Autodesk Inventor part; units mm, degrees
ref_plane "YZ Plane" through (0, 0, 0) normal (1, 0, 0) x (0, 1, 0)
ref_plane "XZ Plane" through (0, 0, 0) normal (0, 1, 0) x (-1, 0, 0)
ref_plane "XY Plane" through (0, 0, 0) normal (0, 0, 1) x (1, 0, 0)
sketch "Sketch1" plane through (0, 0, 0) normal (0, 0, 1) x (1, 0, 0)
  circle A0 centre (0, 0) radius 6.35
  line L0 (0, 10.9985) -> (9.525, 5.4993)
  line L1 (9.525, 5.4993) -> (9.525, -5.4993)
  line L2 (9.525, -5.4993) -> (0, -10.9985)
  line L3 (0, -10.9985) -> (-9.525, -5.4993)
  line L4 (-9.525, -5.4993) -> (-9.525, 5.4993)
  line L5 (-9.525, 5.4993) -> (0, 10.9985)
  dimension "d1" = 19.05
extrude "Extrusion1" add sketch "Sketch1" against normal blind 12.7 contours A0 | L0 L1 L2 L3 L4 L5
sketch "Sketch2" plane through (0, 0, 0) normal (0, 0, 1) x (1, 0, 0)
  circle A0 centre (0, 0) radius 6.35
  dimension "d4" = 12.7
extrude "Extrusion2" add sketch "Sketch2" along normal blind 133.35
thread "Thread1"
properties part number "5.25 in bolt"
Can you work these out from the model? Positions are in its coordinate system, mm. A direction names the side the tool comes from. Give positions to 0.01 mm unless a question says otherwise; leave off trailing zeros. Order: outer loops, then holes, each group sorted by start corner. A loop starts at its lowest first (then second) coordinate and runs counter-clockwise, first axis right, second up. Notation, with made-up numbers: M -32,-32.75 L 9,-32.75 A29 cw 9,4.25 Z; hole C 74,78.5 d1. An arc over 180 degrees is marked long. Use a Markdown table: item, result. Add a question column.
Item 1: Suppose I cut it at B-B (x = 4). List the corners of the cut face in (y, z) for me.
Item 2: For faces 1 (the cylindrical face through (-1.38, 6.2, 65.74)), 2 (the flat face through (0, 0, -12.7)), which set-ups out of +Z, -Z, +X, -X, +Y, -Y let a thin tool reach every point of the face, with its end or its side?
Item 3: If I drill on L1, parallel to Z at x = -8.5, y = 5; L2, parallel to X at y = 2.75, z = 13.5; L3, parallel to X at y = 3.75, z = 84, over which ranges is the centre line in solid material (lowest first)? Write a range as [from, to].
Item 4: Will these pins go through, and if not, where does the flat tip stop? pin 1 (5 mm diameter, centred on x = -6.5, z = 19.5, fed in from -Y); pin 2 (6 mm diameter, centred on y = 5, z = 84.5, fed in from -X); pin 3 (2 mm diameter, centred on x = 4.5, z = 31.5, fed in from +Y).
Item 5: Suppose I cut it at C-C (z = 78). List the corners of the cut face in (x, y) for me.
Item 6: Suppose I cut it at A-A (y = 0). List the corners of the cut face in (x, z) for me (3 decimals), then the cut area to 3 significant figures.
Answer sheet:
| question | item | result |
|---|---|---|
| 1 | outline | M -8.69,-12.7 L 8.69,-12.7 L 8.69,0 L 4.93,0 L 4.93,133.35 L -4.93,133.35 L -4.93,0 L -8.69,0 Z |
| 2 | face 1 | +Z |
| 2 | face 2 | -Z, +X, -X, +Y, -Y |
| 3 | L1 | z = [-12.7, 0] |
| 3 | L2 | x = [-5.72, 5.72] |
| 3 | L3 | x = [-5.12, 5.12] |
| 4 | pin 1 | stops at y = -4.93 |
| 4 | pin 2 | stops at x = -6.03 |
| 4 | pin 3 | stops at y = 5.3 |
| 5 | outline | C 0,0 d12.7 |
| 6 | outline | M -9.525,-12.7 L 9.525,-12.7 L 9.525,0 L 6.35,0 L 6.35,133.35 L -6.35,133.35 L -6.35,0 L -9.525,0 Z |
| 6 | area | 1,940 mm² |
